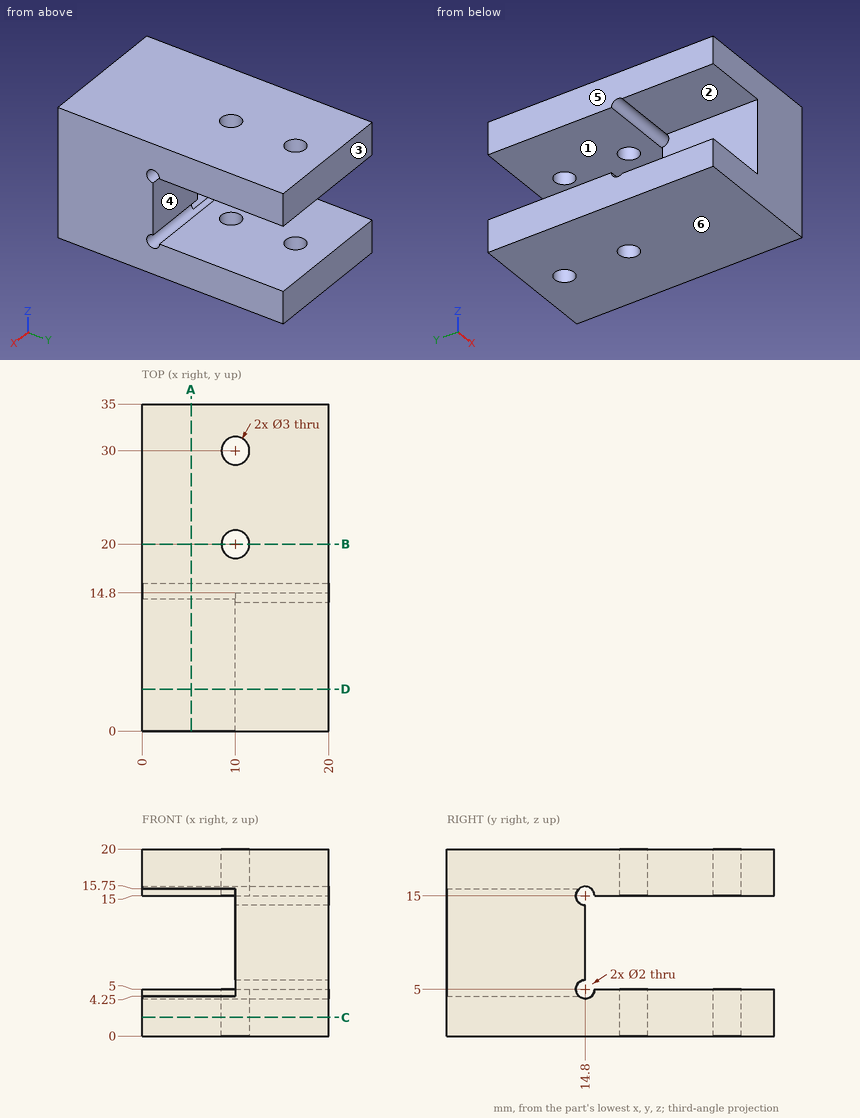
Design review of the part shown in the three views and the two pictorial views. Dimensions are in mm from the part's minimum x, y and z. A direction names the side the tool comes from. Give positions to 0.01 mm unless a question says otherwise; leave off trailing zeros. Loops run counter-clockwise (first coordinate to the right, second up) from the corner with the lowest first, then second, coordinate; pieces in that order, holes last. Notation, with made-up numbers: (12, 60.5) -> (69, 60.5) arc R19 ccw to (69, 72.5) -> close; hole circle Ø2 at (-27.5, 5). An arc over 180 degrees is marked (long way). Answer as a JSON object with one key per item and string values. Group by question number.
Q1. Tool access review of the marked faces 1, 2 and 3: name each direction out of +Z, -Z, +X, -X, +Y, -Y from which nothing blocks a thin tool from reaching the whole face with its end or side.
Q2. Take a section at C-C (z = 2). Write out the cut boundary in (x, y).
Q3. Insertion check: pin 1 (2.5 mm diameter, centred on x = 10, y = 30, fed in from -Z); pin 2 (9 mm diameter, centred on y = 7, z = 9, fed in from -X); pin 3 (4 mm diameter, centred on x = 15.5, z = 10.5, fed in from +Y). Each pin has a flat end and moves straight along its axis. Give the tip position at first contact, or say it passes through.
Q4. Wall thickness on line 1 along Y through (x, z) = (10, 17.2); line 2 along Z through (x, y) = (7.5, 19.5); line 3 along Z through (x, y) = (2.5, 12): over which ranges is each line inside the solid? List them lowest first.
Q5. Take a section at B-B (y = 20). Write out the cut boundary in (x, z).
Q6. Take a section at D-D (y = 4.5). Write out the cut boundary in (x, z).
Q7. Take a section at A-A (x = 5.25). Write out the cut boundary in (y, z).
Q8. Draft analysis for pull direction Z (two halves, no side actions). For the marked faces 4, 5 and 6, state which applies: pulls with the +Z half, pulls with the -Z half, needs draft (parallel to the pull), parting line crosses it, or undercut.
Answer below:
{
 "1": {"face 1": "+X, -X, +Y", "face 2": "-X, -Y", "face 3": "+Z, -Z, +X, -X, +Y"},
 "2": {"outline": "(0, 0) -> (20, 0) -> (20, 35) -> (0, 35) -> close; hole circle Ø3 at (10, 20); hole circle Ø3 at (10, 30)"},
 "3": {"pin 1": "passes through", "pin 2": "stops at x = 10", "pin 3": "stops at y = 14.8"},
 "4": {"line 1": "y = 0 to 18.5, 21.5 to 28.5, 31.5 to 35", "line 2": "z = 0 to 5, 15 to 20", "line 3": "z = 0 to 4.25, 15.75 to 20"},
 "5": {"outline": "(0, 0) -> (8.5, 0) -> (8.5, 5) -> (0, 5) -> close; (0, 15) -> (8.5, 15) -> (8.5, 20) -> (0, 20) -> close; (11.5, 0) -> (20, 0) -> (20, 5) -> (11.5, 5) -> close; (11.5, 15) -> (20, 15) -> (20, 20) -> (11.5, 20) -> close"},
 "6": {"outline": "(0, 0) -> (20, 0) -> (20, 20) -> (0, 20) -> (0, 15.75) -> (10, 15.75) -> (10, 4.25) -> (0, 4.25) -> close"},
 "7": {"outline": "(0, 0) -> (35, 0) -> (35, 5) -> (15.8, 5) arc R1 cw to (14.14, 4.25) -> (0, 4.25) -> close; (0, 15.75) -> (14.14, 15.75) arc R1 cw to (15.8, 15) -> (35, 15) -> (35, 20) -> (0, 20) -> close"},
 "8": {"face 4": "undercut", "face 5": "needs draft", "face 6": "pulls with the -Z half"}
}
